```python
from build123d import *

# Parameters (mm, degrees)
SKETCH1_R           = 7.5
BOSS_EXTRUDE1_DEPTH = 5


with BuildPart() as part:
    # Sketch1 → Boss-Extrude1 (new, symmetric)
    with BuildSketch(Plane.XY):
        with BuildLine():
            ThreePointArc((31.620603921, 7.494504901), (17.82100855, 16.145486471), (1.973178454, 19.902426153))
            ThreePointArc((1.973178454, 19.902426153), (0.987071189, 19.960959504), (0, 20))
            ThreePointArc((0, 20), (-20, 0), (0, -20))
            ThreePointArc((0, -20), (0.987071189, -19.960959504), (1.973178454, -19.902426153))
            ThreePointArc((1.973178454, -19.902426153), (17.82100855, -16.145486471), (31.620603921, -7.494504901))
            ThreePointArc((31.620603921, -7.494504901), (35, 0), (31.620603921, 7.494504901))
        make_face()
        Circle(SKETCH1_R, mode=Mode.SUBTRACT)
    extrude(amount=BOSS_EXTRUDE1_DEPTH, both=True)


solid = part.part
```
Source: CAD feature listing. Evaluate the final solid. Frame: model axes, mm. Round coordinates to 2 decimals unless told otherwise and drop trailing zeros. Write each loop counter-clockwise with the first axis right and the second up, starting at its lowest first coordinate (ties: lowest second). Pieces come first, ordered by that corner, then holes. Notation, with made-up numbers: M 58.25,-33 L 97.25,-33 A7 ccw 97.25,-21 Z; hole C -23.5,19.25 d9. An arc over 180 degrees is marked long. Answer as a JSON object with one key per item and string values. Group by question number.
(1) Section query C-C on x = -4. Output: boundary loops of the cut face in (y, z).
(2) Section query B-B on z = 0.25. Output: boundary loops of the cut face in (x, y), then the cut area to 3 significant figures.
(3) Ray query, line 1 (Y direction, x = 0, z = -2); line 2 (X direction, y = -4, z = -3.75); line 3 (X direction, y = -3, z = 3.75). Return the intervals inside material, ascending. Write a range as [from, to].
(4) Section query A-A on y = 0. Output: boundary loops of the cut face in (x, z), then the cut area to 3 significant figures.
(5) Section query D-D on y = -13. Output: boundary loops of the cut face in (x, z), then the cut area to 3 significant figures.
(6) First-contact query: pin 1 (5 mm diameter, centred on x = 17, z = 1, fed in from -Y); pin 2 (1.5 mm diameter, centred on y = 10, z = -3.5, fed in from -X); pin 3 (5 mm diameter, centred on x = 5, z = 1, fed in from +Y); pin 4 (13.5 mm diameter, centred on x = 0, y = 0, fed in from -Z). Flat tips, straight axial feed; report the tip coordinate or a pass-through.
(7) Mould query, pull axis X, two halves, no side actions, for faces 1 (the flat face through (7, -4, 5)), 2 (the cylindrical face through (-7.493, 0.33, -0.07)), 3 (the cylindrical face through (-20, 0, 0)). Classes: +X half, -X half, draft (parallel to the pull), parting line (faces both ways), or undercut.
Computed values:
{
 "1": {"outline": "M -19.6,-5 L -6.34,-5 L -6.34,5 L -19.6,5 Z; M 6.34,-5 L 19.6,-5 L 19.6,5 L 6.34,5 Z"},
 "2": {"outline": "M 0,-20 A50 ccw 31.62,-7.49 A10 ccw 31.62,7.49 A50 ccw 0,20 A20 ccw Z; hole C 0,0 d15", "area": "1,490 mm^2"},
 "3": {"line 1": "[-20, -7.5], [7.5, 20]", "line 2": "[-19.6, -6.34], [6.34, 34.17]", "line 3": "[-19.77, -6.87], [6.87, 34.54]"},
 "4": {"outline": "M -20,-5 L -7.5,-5 L -7.5,5 L -20,5 Z; M 7.5,-5 L 35,-5 L 35,5 L 7.5,5 Z", "area": "400 mm^2"},
 "5": {"outline": "M -15.2,-5 L 24.07,-5 L 24.07,5 L -15.2,5 Z", "area": "393 mm^2"},
 "6": {"pin 1": "y = -17.4", "pin 2": "x = -17.73", "pin 3": "y = 19.86", "pin 4": "through"},
 "7": {"face 1": "draft", "face 2": "undercut", "face 3": "-X half"}
}
